from build123d import *

# Parameters (mm, degrees)
SKETCH2_W                  = 78.5
SKETCH2_H                  = 50.4
BOSS_EXTRUDE2_DEPTH        = 10
SKETCH3_W                  = 68.5
SKETCH3_H                  = 40.4
CUT_EXTRUDE1_DEPTH         = 5
SKETCH6_W                  = 33.6
SKETCH6_H                  = 33.6
SKETCH6_R                  = 11.8
BOSS_EXTRUDE4_DEPTH        = 10
M6X1_0_TAPPED_HOLE5_REACH  = 90.653
M6X1_0_TAPPED_HOLE5_BORE_R = 2.5


with BuildPart() as part:
    # Sketch2 → Boss-Extrude2 (new body)
    with BuildSketch(Plane(origin=(0, 0, 0), x_dir=(1, 0, 0), z_dir=(0, 1, 0))):
        with Locations((-42.320258308, 20.202024982)):
            Rectangle(SKETCH2_W, SKETCH2_H)
    extrude(amount=BOSS_EXTRUDE2_DEPTH)

    # Sketch3 → Cut-Extrude1 (cut)
    with BuildSketch(Plane(origin=(0, 10, 0), x_dir=(1, 0, 0), z_dir=(0, 1, 0))):
        with Locations((-42.320258308, 20.202024982)):
            Rectangle(SKETCH3_W, SKETCH3_H)
    extrude(amount=-CUT_EXTRUDE1_DEPTH, mode=Mode.SUBTRACT)

    # Sketch6 → Boss-Extrude4 (add)
    with BuildSketch(Plane(origin=(0, 10, 0), x_dir=(1, 0, 0), z_dir=(0, 1, 0))):
        with Locations((-42.320258308, -16.797975018)):
            Rectangle(SKETCH6_W, SKETCH6_H)
        with Locations(Location((-42.320258308, -16.797975018, 0), (0, 0, 270))):
            Circle(SKETCH6_R, mode=Mode.SUBTRACT)
    extrude(amount=-BOSS_EXTRUDE4_DEPTH)

    # M6x1.0 Tapped Hole5 bore (on position points) → M6x1.0 Tapped Hole5 (cut, up to next)
    with BuildSketch(Plane(origin=(-41.704543892, 5.39331072, 33.597975018), x_dir=(1, 0, 0), z_dir=(0, 0, 1)), mode=Mode.PRIVATE) as m6x1_0_tapped_hole5_sk1:
        Circle(M6X1_0_TAPPED_HOLE5_BORE_R)
    m6x1_0_tapped_hole5_tool1 = extrude(m6x1_0_tapped_hole5_sk1.sketch, amount=-M6X1_0_TAPPED_HOLE5_REACH, mode=Mode.PRIVATE) & part.part
    add(m6x1_0_tapped_hole5_tool1.solids().sort_by_distance((-41.704544, 5.393311, 33.597975))[0], mode=Mode.SUBTRACT)


solid = part.part
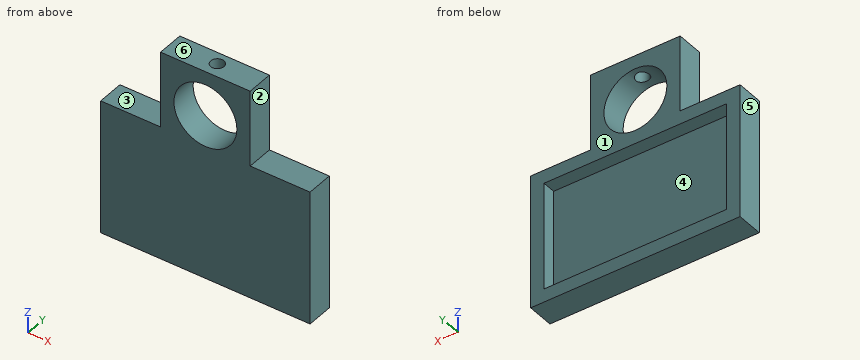
For this review, take the finished solid that the model builds, in its own axes (mm). Face numbers are marked on the shaded views. A direction names the side the tool comes from. Give positions to 0.01 mm unless a question says otherwise; leave off trailing zeros. Order: outer loops, then holes, each group sorted by start corner. A loop starts at its lowest first (then second) coordinate and runs counter-clockwise, first axis right, second up. Notation, with made-up numbers: M 57,23.25 L 95,23.25 A21 cw 95,32.25 Z; hole C 86.5,74.25 d5. An arc over 180 degrees is marked long. Answer in a Markdown table with one row per item. Add a question column.
(1) For pin 1 (2 mm diameter, centred on x = -43, z = -34.5, fed in from +Y); pin 2 (5 mm diameter, centred on y = 4.5, z = 22.5, fed in from -X); pin 3 (3 mm diameter, centred on x = -74, y = 3, fed in from +Z), all flat-tipped, find the tip position at first contact; note any pin that passes through.
(2) Wall thickness on probe 1 along X at (y, z) = (7.25, -32); probe 2 along Z at (x, y) = (-75, 7.25); probe 3 along Z at (x, y) = (-58.5, 9): over which ranges is each line inside the solid? List them lowest first. Write a range as [from, to].
(3) Consider section C-C on y = 6.75. State the section outline as (x, z) points, and give its area (3 significant figures).
(4) For the marked faces 1, 2 and 3, list the 3-axis set-ups (+Z, -Z, +X, -X, +Y, -Y) from which the entire face can be reached by the end or side of a thin tool; tool diameter is ignored.
(5) Mouldability with a two-part tool opening along X and no side actions: class the marked faces 4, 5 and 6 as +X half, -X half, draft (parallel to the pull), parting line (faces both ways), or undercut.
(6) Consider section B-B on x = -32.5. State the section outline as (y, z) points.
(7) Consider section A-A on z = 13.5. State the section outline as (x, y) points, and give its area (3 significant figures).
(8) Consider section D-D on z = -29. State the section outline as (x, y) points, and give its area (4 significant figures).
Evaluation:
| question | item | result |
|---|---|---|
| 1 | pin 1 | stops at y = 5 |
| 1 | pin 2 | stops at x = -59.12 |
| 1 | pin 3 | stops at z = 5 |
| 2 | probe 1 | x = [-81.57, -76.57], [-8.07, -3.07] |
| 2 | probe 2 | z = [-45.4, -40.4], [0, 5] |
| 2 | probe 3 | z = [-45.4, -40.4], [0, 33.6] |
| 3 | outline | M -81.57,-45.4 L -3.07,-45.4 L -3.07,5 L -25.52,5 L -25.52,33.6 L -39.6,33.6 L -39.6,28.28 A11.8 cw long -43.8,28.5 L -43.8,33.6 L -59.12,33.6 L -59.12,5 L -81.57,5 Z; hole M -76.57,-40.4 L -8.07,-40.4 L -8.07,0 L -76.57,0 Z |
| 3 | area | 1,690 mm^2 |
| 4 | face 1 | +Z, -Z, +X, -X, +Y |
| 4 | face 2 | +Z, +X, +Y, -Y |
| 4 | face 3 | +Z, -X, +Y, -Y |
| 5 | face 4 | undercut |
| 5 | face 5 | -X half |
| 5 | face 6 | draft |
| 6 | outline | M 0,-45.4 L 10,-45.4 L 10,-40.4 L 5,-40.4 L 5,0 L 10,0 L 10,10.26 L 0,10.26 Z; M 0,23.34 L 10,23.34 L 10,33.6 L 0,33.6 Z |
| 7 | outline | M -59.12,0 L -53.65,0 L -53.65,10 L -59.12,10 Z; M -30.99,0 L -25.52,0 L -25.52,10 L -30.99,10 Z |
| 7 | area | 109 mm^2 |
| 8 | outline | M -81.57,0 L -3.07,0 L -3.07,10 L -8.07,10 L -8.07,5 L -76.57,5 L -76.57,10 L -81.57,10 Z |
| 8 | area | 442.5 mm^2 |
